Verification items for the finished model (mm, model axes). Face numbers are marked on the shaded views. A direction names the side the tool comes from. Give positions to 0.01 mm unless a question says otherwise; leave off trailing zeros. Loops run counter-clockwise (first coordinate to the right, second up) from the corner with the lowest first, then second, coordinate; pieces in that order, holes last. Notation, with made-up numbers: (-34, -39.5) -> (14, -39.5) arc R23 ccw to (14, -24.5) -> close; hole circle Ø10 at (59.5, -33.5). An arc over 180 degrees is marked (long way). Use one line per item in the form item = value. Start each with the question number.
from build123d import *

# Parameters (mm, degrees)
F2_R     = 2.5
F3_DEPTH = 25
F4_R     = 20
F4_R_2   = 15
F4_R_3   = 2.5
F5_DEPTH = 5
F6_DEPTH = 5


with BuildPart() as f1:
    # F0 (on Front) → F1 (revolve)
    with BuildSketch(Plane.XZ):
        with BuildLine():
            Line((0, 0), (0, 5))
            add(Edge.make_bspline(
                [(0, 5), (-15, 5), (-15, 0)],
                knots=[4.7123889804, 4.7123889804, 4.7123889804, 6.2831853072, 6.2831853072, 6.2831853072], degree=2, weights=[1, 0.7071067812, 1]))
            Line((-15, 0), (0, 0))
        make_face()
    revolve(axis=Axis((0, 0, 2.5), (0, 0, 1)))

    # F2 (on face) → F3 (cut)
    with BuildSketch(Plane(origin=(0, 0, 0), x_dir=(1, 0, 0), z_dir=(0, 0, -1))):
        with Locations((5.9301354922, -6.6626928747)):
            Circle(F2_R)
        with BuildLine():
            ThreePointArc((-5.2131647244, 2.2031189874), (-3.1274667568, 4.7169663346), (0, 5.6595776977))
            ThreePointArc((0, 5.6595776977), (3.1274667568, 4.7169663346), (5.2131647244, 2.2031189874))
            ThreePointArc((5.2131647244, 2.2031189874), (8.4891528404, 0.8734942796), (9.8187775482, 4.1494823956))
            ThreePointArc((9.8187775482, 4.1494823956), (5.8904527284, 8.8842086506), (0, 10.6595776977))
            ThreePointArc((0, 10.6595776977), (-5.8904527284, 8.8842086506), (-9.8187775482, 4.1494823956))
            ThreePointArc((-9.8187775482, 4.1494823956), (-8.4891528404, 0.8734942796), (-5.2131647244, 2.2031189874))
        make_face()
        with Locations((-5.9301354922, -6.6626928747)):
            Circle(F2_R)
    extrude(amount=-F3_DEPTH, mode=Mode.SUBTRACT)

    # F4 (on face) → F5 (join)
    with BuildSketch(Plane(origin=(0, 0, 0), x_dir=(1, 0, 0), z_dir=(0, 0, -1))):
        Polygon((-25, -25), (0, -25), (25, -25), (25, 0), (25, 25), (0, 25), (-25, 25), (-25, 0), align=None)
        Circle(F4_R, mode=Mode.SUBTRACT)
        Circle(F4_R)
        Circle(F4_R_2, mode=Mode.SUBTRACT)
        Circle(F4_R_2)
        with Locations((-5.9301354922, -6.6626928747)):
            Circle(F4_R_3, mode=Mode.SUBTRACT)
        with Locations((5.9301354922, -6.6626928747)):
            Circle(F4_R_3, mode=Mode.SUBTRACT)
        with BuildLine():
            ThreePointArc((-5.2131647244, 2.2031189874), (-8.4891528404, 0.8734942796), (-9.8187775482, 4.1494823956))
            ThreePointArc((-9.8187775482, 4.1494823956), (0, 10.6595776977), (9.8187775482, 4.1494823956))
            ThreePointArc((9.8187775482, 4.1494823956), (8.4891528404, 0.8734942796), (5.2131647244, 2.2031189874))
            ThreePointArc((5.2131647244, 2.2031189874), (0, 5.6595776977), (-5.2131647244, 2.2031189874))
        make_face(mode=Mode.SUBTRACT)
        with BuildLine():
            ThreePointArc((9.8187775482, 4.1494823956), (0, 10.6595776977), (-9.8187775482, 4.1494823956))
            ThreePointArc((-9.8187775482, 4.1494823956), (-8.4891528404, 0.8734942796), (-5.2131647244, 2.2031189874))
            ThreePointArc((-5.2131647244, 2.2031189874), (0, 5.6595776977), (5.2131647244, 2.2031189874))
            ThreePointArc((5.2131647244, 2.2031189874), (8.4891528404, 0.8734942796), (9.8187775482, 4.1494823956))
        make_face()
        with Locations((5.9301354922, -6.6626928747)):
            Circle(F4_R_3)
        with Locations((-5.9301354922, -6.6626928747)):
            Circle(F4_R_3)
    extrude(amount=F5_DEPTH)

    # F4 (on face) → F6 (join)
    with BuildSketch(Plane(origin=(0, 0, 0), x_dir=(1, 0, 0), z_dir=(0, 0, -1))):
        Polygon((-25, -25), (0, -25), (25, -25), (25, 0), (25, 25), (0, 25), (-25, 25), (-25, 0), align=None)
        Circle(F4_R, mode=Mode.SUBTRACT)
    extrude(amount=-F6_DEPTH)


solid = f1.part
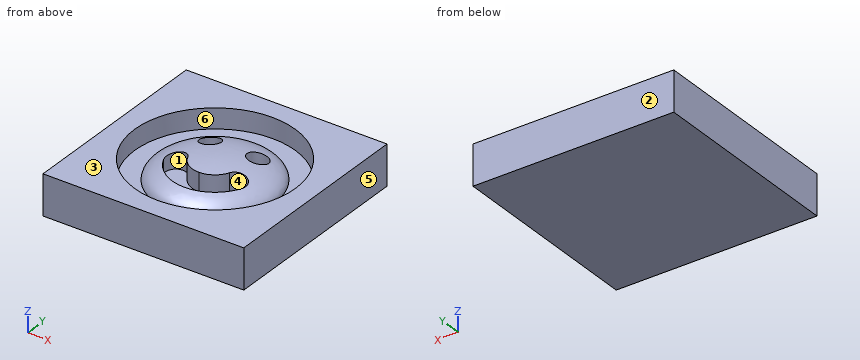
Item 1: Gauge pin test, flat ends, axial feed: pin 1 Ø3 at (x, y) = (4, -7) entering from +Z; pin 2 Ø6 at (x, y) = (7.5, -1.5) entering from +Z; pin 3 Ø2 at (x, y) = (6.5, -11.5) entering from +Z. Record the tip position at first contact, or that the pin passes through.
Item 2: Draft check along X on the marked faces 3, 4, 5 and 6. Enter one of: +X half, -X half, draft (parallel to the pull), parting line (faces both ways), or undercut.
Item 3: Tool access check on the marked faces 1 and 2. Record the directions out of +Z, -Z, +X, -X, +Y, -Y that give a thin tool (end or side, any length) a straight path to the whole face; none if there is none.
Item 4: Sectioned sample at A-A, the plane x = 18.5. Enter the section's corners in (y, z), and give its area (3 significant figures).
Item 5: Material ranges on line 1 (Y direction, x = -4, z = 2.25); line 2 (X direction, y = 10, z = 1.25); line 3 (X direction, y = 0.5, z = 1.75), recorded low to high.
Outcome:
q1.pin_1 = 0
q1.pin_2 = 4.75
q1.pin_3 = 2.9
q2.face_3 = draft
q2.face_4 = undercut
q2.face_5 = +X half
q2.face_6 = undercut
q3.face_1 = +Z
q3.face_2 = +Z, -Z, +X, -X, +Y
q4.outline = (-25, -5) -> (25, -5) -> (25, 5) -> (7.6, 5) -> (7.6, 0) -> (-7.6, 0) -> (-7.6, 5) -> (-25, 5) -> close
q4.area = 424 mm^2
q5.line_1 = -25 to -19.6, -12.78 to -9.88, -4 to 5.07, 8.25 to 12.78, 19.6 to 25
q5.line_2 = -25 to -17.32, -10.53 to 10.53, 17.32 to 25
q5.line_3 = -25 to -19.99, -14.04 to 14.04, 19.99 to 25
